Could you check a few things on this model? Use its own coordinates, in mm. Coordinates: 2 decimals unless noted, no trailing zeros. Order: outer loops, then holes, each group sorted by start corner. A loop starts at its lowest first (then second) coordinate and runs counter-clockwise, first axis right, second up. Notation, with made-up numbers: (46.25, 69) -> (59.25, 69) arc R21 cw to (59.25, 81) -> close; hole circle Ø10 at (47.25, 67). An arc over 180 degrees is marked (long way). Use a Markdown table: item, result. Add a question column.
1) If I drill on L1, parallel to Y at x = 18.5, z = -8; L2, parallel to Z at x = 35, y = 586.4; L3, parallel to Z at x = 6.5, y = 454, over which ranges is the centre line in solid material (lowest first)? Write a range as [from, to].
2) If we section it at B-B (y = 128.5): Write out the boundary of the cut face in (x, z), plus the area to 3 significant figures.
3) Thinking about a two-plate mould opening in Y: for faces 1 (the flat face through (-1, 0, -7)), 2 (the cylindrical face through (45, -1, 0)), 3 (the flat face through (-1, 587, 0)), which applies, +Y half, -Y half, draft (parallel to the pull), parting line (faces both ways), or undercut?
4) Will these pins go through, and if not, where does the flat tip stop? pin 1 Ø4 at (y, z) = (373, -2.5) entering from -X; pin 2 Ø4.5 at (x, z) = (35, 0) entering from +Y; pin 3 Ø6 at (y, z) = (211.5, 6.5) entering from -X.
5) If we section it at A-A (x = 24): Write out the boundary of the cut face in (y, z), plus the area to 3 significant figures.
```python
from build123d import *

# Parameters (mm, degrees)
F1_R     = 2.5
F2_DEPTH = 3
F4_DEPTH = 292


with BuildPart() as f2:
    # F1 (on Front) → F2 (new body)
    with BuildSketch(Plane.XZ):
        with BuildLine():
            ThreePointArc((35, -10), (45, 0), (35, 10))
            Line((35, 10), (0, 10))
            Line((0, 10), (-35, 10))
            ThreePointArc((-35, 10), (-45, 0), (-35, -10))
            Line((-35, -10), (0, -10))
            Line((0, -10), (35, -10))
        make_face()
        with Locations((-35, 0)):
            Circle(F1_R, mode=Mode.SUBTRACT)
        with Locations((35, 0)):
            Circle(F1_R, mode=Mode.SUBTRACT)
    extrude(amount=F2_DEPTH)

    # F3 (on face) → F4 (join, through all)
    with BuildSketch(Plane(origin=(0, 0, 0), x_dir=(-1, 0, 0), z_dir=(0, 1, 0))):
        Polygon((7.071068, 0), (0, 7.071068), (-7.071068, 0), (0, -7.071068), align=None)
    extrude(amount=F4_DEPTH)

    # F5: F2 across plane


with BuildPart() as f2_1:
    add(f2.part)
    add(f2.part.mirror(Plane.XZ.offset(-292)))


solid = f2_1.part
```
Answer sheet:
| question | item | result |
|---|---|---|
| 1 | L1 | [-3, 0], [584, 587] |
| 1 | L2 | [-10, -2.5], [2.5, 10] |
| 1 | L3 | [-0.57, 0.57] |
| 2 | outline | (-7.07, 0) -> (0, -7.07) -> (7.07, 0) -> (0, 7.07) -> close |
| 2 | area | 100 mm2 |
| 3 | face 1 | undercut |
| 3 | face 2 | draft |
| 3 | face 3 | +Y half |
| 4 | pin 1 | x = -6.57 |
| 4 | pin 2 | through |
| 4 | pin 3 | x = -3.57 |
| 5 | outline | (-3, -10) -> (0, -10) -> (0, 10) -> (-3, 10) -> close; (584, -10) -> (587, -10) -> (587, 10) -> (584, 10) -> close |
| 5 | area | 120 mm2 |
